from build123d import *


with BuildPart() as part:
    # Esquisse1 → Révolution1 (revolve)
    with BuildSketch(Plane.XY):
        with BuildLine():
            Line((11.5, 1.406527307), (11.5, -8.206711775))
            Line((11.5, -8.206711775), (8, -12.301381653))
            Line((8, -12.301381653), (8, -17.475))
            Line((8, -17.475), (3, -17.475))
            Line((3, -17.475), (3, -31.475))
            Line((3, -31.475), (0, -31.475))
            Line((0, -31.475), (0, 9.525))
            ThreePointArc((0, 9.525), (4.879805324, 8.180044315), (8.381527307, 4.525))
            ThreePointArc((8.381527307, 4.525), (10.586620495, 3.611620495), (11.5, 1.406527307))
        make_face()
    revolve(axis=Axis((0, 9.525, 0), (0, -1, 0)))


solid = part.part
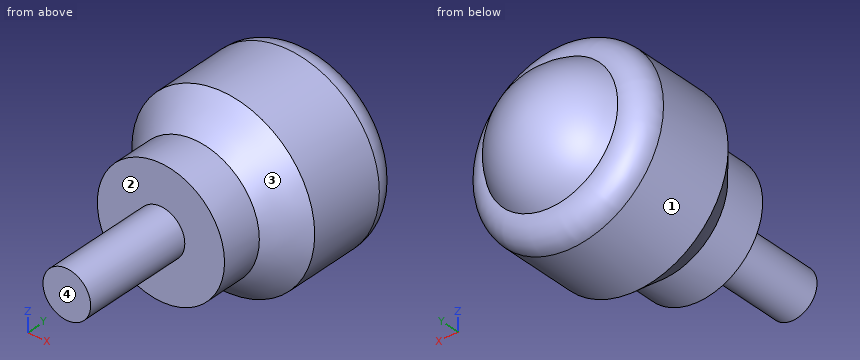
The model under review builds one solid part; all positions refer to its coordinate system, in mm. Face numbers are marked on the shaded views. A direction names the side the tool comes from. Round coordinates to 2 decimals unless told otherwise and drop trailing zeros. Loops run counter-clockwise (first coordinate to the right, second up) from the corner with the lowest first, then second, coordinate; pieces in that order, holes last. Notation, with made-up numbers: (-9, 45) -> (28, 45) arc R23 ccw to (28, 61) -> close; hole circle Ø7 at (34, 65.5). An arc over 180 degrees is marked (long way). One line per question, with ' | ' between items. Start each with the question number.
Item 1: Add section A-A, the plane z = 0. Write out the cut boundary in (x, y) (3 decimals), then the cut area to 3 significant figures.
Item 2: Machinability: for the marked faces 1 and 2, which of the approach directions +Z, -Z, +X, -X, +Y, -Y give a long, thin tool a straight path to every point of the face, cutting with its end or side? Answer none if there is none.
Item 3: Add section C-C, the plane y = -16. Write out the cut boundary in (x, z).
Item 4: Add section D-D, the plane y = -28.5. Write out the cut boundary in (x, z).
Item 5: Add section B-B, the plane x = 0. Write out the cut boundary in (y, z) (3 decimals).
Item 6: Wall thickness on line 1 along Z through (x, y) = (8.25, -8); line 2 along Z through (x, y) = (4.5, -14); line 3 along Y through (x, z) = (-1.75, -7) (3 decimals): over which ranges is each line inside the solid? List them lowest first. Write a range as [from, to].
Item 7: For pin 1 (1.5 mm diameter, centred on y = -15.5, z = 6, fed in from -X); pin 2 (12 mm diameter, centred on y = -17, z = -7.5, fed in from +X); pin 3 (2 mm diameter, centred on x = -5.5, y = -9, fed in from +Z), all flat-tipped, find the tip position at first contact; note any pin that passes through.
Item 8: Draft analysis for pull direction X (two halves, no side actions). For the marked faces 3 and 4, state which applies: +X half, -X half, draft (parallel to the pull), parting line (faces both ways), or undercut.
Return value:
1) outline: (-11.5, -8.207) -> (-8, -12.301) -> (-8, -17.475) -> (-3, -17.475) -> (-3, -31.475) -> (3, -31.475) -> (3, -17.475) -> (8, -17.475) -> (8, -12.301) -> (11.5, -8.207) -> (11.5, 1.407) arc R3.118 ccw to (8.382, 4.525) arc R9.525 ccw to (-8.382, 4.525) arc R3.118 ccw to (-11.5, 1.407) -> close | area: 595 mm2
2) face 1: +Y, -Y | face 2: -Y
3) outline: circle Ø16 at (0, 0)
4) outline: circle Ø6 at (0, 0)
5) outline: (-31.475, -3) -> (-17.475, -3) -> (-17.475, -8) -> (-12.301, -8) -> (-8.207, -11.5) -> (1.407, -11.5) arc R3.118 ccw to (4.525, -8.382) arc R9.525 ccw to (4.525, 8.382) arc R3.118 ccw to (1.407, 11.5) -> (-8.207, 11.5) -> (-12.301, 8) -> (-17.475, 8) -> (-17.475, 3) -> (-31.475, 3) -> close
6) line 1: z = [-8.01, 8.01] | line 2: z = [-6.61, 6.61] | line 3: y = [-17.475, 6.218]
7) pin 1: stops at x = -6.04 | pin 2: stops at x = 7.86 | pin 3: stops at z = 10.41
8) face 3: parting line | face 4: draft
